Autodesk Inventor part; units mm, degrees
ref_plane "YZ Plane" through (0, 0, 0) normal (1, 0, 0) x (0, 1, 0)
ref_plane "XZ Plane" through (0, 0, 0) normal (0, 1, 0) x (-1, 0, 0)
ref_plane "XY Plane" through (0, 0, 0) normal (0, 0, 1) x (1, 0, 0)
sketch "Sketch1" plane through (0, 0, 0) normal (0, 0, 1) x (1, 0, 0)
  line L0 (-12.5, 15) -> (12.5, 15)
  line L1 (12.5, 15) -> (12.5, -12)
  line L2 (9.5, -15) -> (-12.5, -15)
  line L3 (-12.5, -15) -> (-12.5, 15)
  line L4 (-12.5, 15) -> (12.5, -15) construction
  line L5 (12.5, 15) -> (-12.5, -15) construction
  line L6 (9.5, -15) -> (12.5, -12)
  point P0 (0, 0)
  dimension "d0" = 25
  dimension "d1" = 30
  dimension "d2" = 3
  dimension "d3" = 3
extrude "Extrusion1" add sketch "Sketch1" along normal blind 1.6
sketch "Sketch2" plane through (0, 0, 1.6) normal (0, 0, 1) x (1, 0, 0)
  line L0 (-4, -3) -> (4, -3)
  line L1 (4, -3) -> (4, -11)
  line L2 (4, -11) -> (-4, -11)
  line L3 (-4, -11) -> (-4, -3)
  line L4 (-4, -3) -> (4, -11) construction
  line L5 (4, -3) -> (-4, -11) construction
  line L6 (-12.5, -15) -> (9.5, -15)
  point P0 (0, 0)
  point P1 (0, -7)
  dimension "d6" = 8
  dimension "d7" = 8
  dimension "d8" = 8
extrude "Extrusion2" add sketch "Sketch2" along normal blind 1.6
sketch "Sketch5" plane through (0, 0, 1.6) normal (0, 0, 1) x (1, 0, 0)
  line L0 (-12.3, 8) -> (-10.5, 8)
  line L1 (-10.5, 8) -> (-10.5, 6.2)
  line L2 (-10.5, 6.2) -> (-12.3, 6.2)
  line L3 (-12.3, 6.2) -> (-12.3, 8)
  line L4 (-12.3, 8) -> (-10.5, 6.2) construction
  line L5 (-10.5, 8) -> (-12.3, 6.2) construction
  line L6 (-12.5, 15) -> (-12.5, -15)
  line L7 (-12.3, 3.66) -> (-12.3, 5.46)
  line L8 (-12.3, 5.46) -> (-10.5, 5.46)
  line L9 (-10.5, 5.46) -> (-10.5, 3.66)
  line L10 (-10.5, 3.66) -> (-12.3, 3.66)
  line L11 (-12.3, 1.12) -> (-12.3, 2.92)
  line L12 (-12.3, 2.92) -> (-10.5, 2.92)
  line L13 (-10.5, 2.92) -> (-10.5, 1.12)
  line L14 (-10.5, 1.12) -> (-12.3, 1.12)
  line L15 (-12.3, -1.42) -> (-12.3, 0.38)
  line L16 (-12.3, 0.38) -> (-10.5, 0.38)
  line L17 (-10.5, 0.38) -> (-10.5, -1.42)
  line L18 (-10.5, -1.42) -> (-12.3, -1.42)
  line L19 (-12.3, -3.96) -> (-12.3, -2.16)
  line L20 (-12.3, -2.16) -> (-10.5, -2.16)
  line L21 (-10.5, -2.16) -> (-10.5, -3.96)
  line L22 (-10.5, -3.96) -> (-12.3, -3.96)
  line L23 (-12.3, -6.5) -> (-12.3, -4.7)
  line L24 (-12.3, -4.7) -> (-10.5, -4.7)
  line L25 (-10.5, -4.7) -> (-10.5, -6.5)
  line L26 (-10.5, -6.5) -> (-12.3, -6.5)
  line L27 (-12.3, -9.04) -> (-12.3, -7.24)
  line L28 (-12.3, -7.24) -> (-10.5, -7.24)
  line L29 (-10.5, -7.24) -> (-10.5, -9.04)
  line L30 (-10.5, -9.04) -> (-12.3, -9.04)
  line L31 (-12.3, -11.58) -> (-12.3, -9.78)
  line L32 (-12.3, -9.78) -> (-10.5, -9.78)
  line L33 (-10.5, -9.78) -> (-10.5, -11.58)
  line L34 (-10.5, -11.58) -> (-12.3, -11.58)
  line L35 (12.5, 15) -> (-12.5, 15)
  line L36 (10.56, 6.2) -> (10.56, 8)
  line L37 (10.56, 8) -> (12.36, 8)
  line L38 (12.36, 8) -> (12.36, 6.2)
  line L39 (12.36, 6.2) -> (10.56, 6.2)
  line L40 (10.56, 3.66) -> (10.56, 5.46)
  line L41 (10.56, 5.46) -> (12.36, 5.46)
  line L42 (12.36, 5.46) -> (12.36, 3.66)
  line L43 (12.36, 3.66) -> (10.56, 3.66)
  line L44 (10.56, 1.12) -> (10.56, 2.92)
  line L45 (10.56, 2.92) -> (12.36, 2.92)
  line L46 (12.36, 2.92) -> (12.36, 1.12)
  line L47 (12.36, 1.12) -> (10.56, 1.12)
  line L48 (10.56, -1.42) -> (10.56, 0.38)
  line L49 (10.56, 0.38) -> (12.36, 0.38)
  line L50 (12.36, 0.38) -> (12.36, -1.42)
  line L51 (12.36, -1.42) -> (10.56, -1.42)
  line L52 (10.56, -3.96) -> (10.56, -2.16)
  line L53 (10.56, -2.16) -> (12.36, -2.16)
  line L54 (12.36, -2.16) -> (12.36, -3.96)
  line L55 (12.36, -3.96) -> (10.56, -3.96)
  line L56 (10.56, -6.5) -> (10.56, -4.7)
  line L57 (10.56, -4.7) -> (12.36, -4.7)
  line L58 (12.36, -4.7) -> (12.36, -6.5)
  line L59 (12.36, -6.5) -> (10.56, -6.5)
  line L60 (10.56, -9.04) -> (10.56, -7.24)
  line L61 (10.56, -7.24) -> (12.36, -7.24)
  line L62 (12.36, -7.24) -> (12.36, -9.04)
  line L63 (12.36, -9.04) -> (10.56, -9.04)
  line L64 (10.56, -11.58) -> (10.56, -9.78)
  line L65 (10.56, -9.78) -> (12.36, -9.78)
  line L66 (12.36, -9.78) -> (12.36, -11.58)
  line L67 (12.36, -11.58) -> (10.56, -11.58)
  point P0 (0, 0)
  point P1 (-11.4, 7.1)
  point P2 (2, 15)
  dimension "d19" = 1.8
  dimension "d20" = 1.8
  dimension "d21" = 1.1
  dimension "d24" = 2.54
  dimension "d29" = 7
  dimension "d32" = 22.86
extrude "Extrusion5" add sketch "Sketch5" along normal blind 0.1
sketch "Sketch6" plane through (-12.5, 15, 0) normal (0, 1, 0) x (1, 0, 0)
  line L0 (19, -3.8) -> (13, -3.8)
  line L1 (13, -3.8) -> (13, 2.2)
  line L2 (13, 2.2) -> (19, 2.2)
  line L3 (19, 2.2) -> (19, -3.8)
  line L4 (19, -3.8) -> (13, 2.2) construction
  line L5 (13, -3.8) -> (19, 2.2) construction
  line L6 (25, 0) -> (25, -1.6)
  point P0 (12.5, 0)
  point P1 (16, -0.8)
  point P2 (25, -0.8)
  dimension "d39" = 6
  dimension "d40" = 6
  dimension "d41" = 6
extrude "Extrusion6" add sketch "Sketch6" along normal blind 2
sketch "Sketch7" plane through (-12.5, 17, 0) normal (0, 1, 0) x (1, 0, 0)
  circle A0 centre (16, -0.8) radius 2.5
  line L0 (13, -3.8) -> (19, -3.8)
  line L1 (13, 2.2) -> (13, -3.8)
  point P0 (12.5, 0)
  point P1 (16, -3.8)
  point P2 (13, -0.8)
  dimension "d44" = 5
extrude "Extrusion7" add sketch "Sketch7" along normal blind 5
equation "\"d3\" = d2"
properties part number "GNSS_board" material "ABS Plastic"
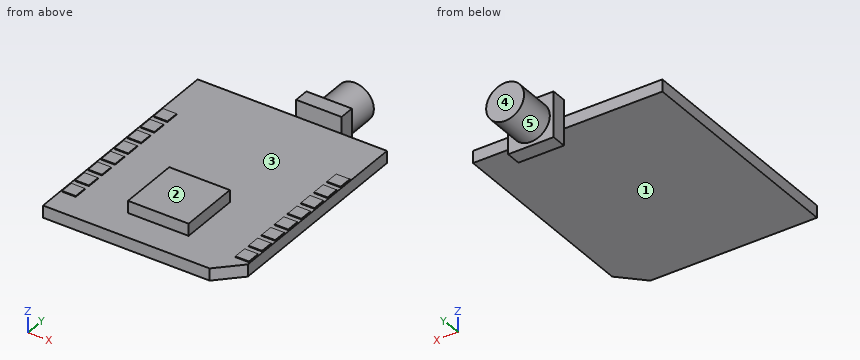
The model under review builds one solid part; all positions refer to its coordinate system, in mm. Face numbers are marked on the shaded views. A direction names the side the tool comes from. Coordinates: 2 decimals unless noted, no trailing zeros. Write each loop counter-clockwise with the first axis right and the second up, starting at its lowest first coordinate (ties: lowest second). Pieces come first, ordered by that corner, then holes. Notation, with made-up numbers: (-38, 37.25) - (6, 37.25) arc R27 cw to (6, 65.25) - close; hole circle Ø2 at (83, 31). An arc over 180 degrees is marked (long way). Answer as a JSON object with one key per item and string values. Group by question number.
1. Add section B-B (x = 3.5). Give the boundary of the cut face in (y, z), plus the area to 3 significant figures.
2. Clearance check with flat-ended pins moving along their axes: pin 1 Ø2 at (x, y) = (-11, 7) entering from +Z; pin 2 Ø12 at (x, y) = (-2, 4) entering from -Z; pin 3 Ø2 at (x, y) = (-6.5, -10.5) entering from +Z. State where each tip first meets the part, or that it passes through.
3. Mouldability with a two-part tool opening along X and no side actions: class the marked faces 3, 4 and 5 as pulls with the +X half, pulls with the -X half, needs draft (parallel to the pull), parting line crosses it, or undercut.
4. Add section A-A (z = 0.8). Give the boundary of the cut face in (x, y), plus the area to 4 significant figures.
5. Add section C-C (y = -0.5). Give the boundary of the cut face in (x, z).
6. Add section D-D (x = -0.75). Give the boundary of the cut face in (y, z).
7. To check wall thickness, follow probe 1 along Y at (x, z) = (-6.75, 1.55); probe 2 along Z at (x, y) = (0.5, -9); probe 3 along Z at (x, y) = (-6.5, 12). State the ranges of each line that lie inside material, in increasing order.
8. Machinability: for the marked faces 1 and 2, which of the approach directions +Z, -Z, +X, -X, +Y, -Y give a long, thin tool a straight path to every point of the face, cutting with its end or side? Answer none if there is none.
Findings:
{
 "1": {"outline": "(-15, 0) - (15, 0) - (15, -2.2) - (17, -2.2) - (17, -1.7) - (22, -1.7) - (22, 3.3) - (17, 3.3) - (17, 3.8) - (15, 3.8) - (15, 1.6) - (-3, 1.6) - (-3, 3.2) - (-11, 3.2) - (-11, 1.6) - (-15, 1.6) - close", "area": "97.8 mm²"},
 "2": {"pin 1": "z = 1.7", "pin 2": "z = 0", "pin 3": "z = 1.6"},
 "3": {"face 3": "undercut", "face 4": "needs draft", "face 5": "parting line crosses it"},
 "4": {"outline": "(-12.5, -15) - (9.5, -15) - (12.5, -12) - (12.5, 15) - (6.5, 15) - (6.5, 17) - (6, 17) - (6, 22) - (1, 22) - (1, 17) - (0.5, 17) - (0.5, 15) - (-12.5, 15) - close", "area": "782.5 mm²"},
 "5": {"outline": "(-12.5, 0) - (12.5, 0) - (12.5, 1.6) - (12.36, 1.6) - (12.36, 1.7) - (10.56, 1.7) - (10.56, 1.6) - (-10.5, 1.6) - (-10.5, 1.7) - (-12.3, 1.7) - (-12.3, 1.6) - (-12.5, 1.6) - close"},
 "6": {"outline": "(-15, 0) - (15, 0) - (15, 1.6) - (-3, 1.6) - (-3, 3.2) - (-11, 3.2) - (-11, 1.6) - (-15, 1.6) - close"},
 "7": {"probe 1": "-15 to 15", "probe 2": "0 to 3.2", "probe 3": "0 to 1.6"},
 "8": {"face 1": "-Z, +X, -X, -Y", "face 2": "+Z, +X, -X, -Y"}
}
